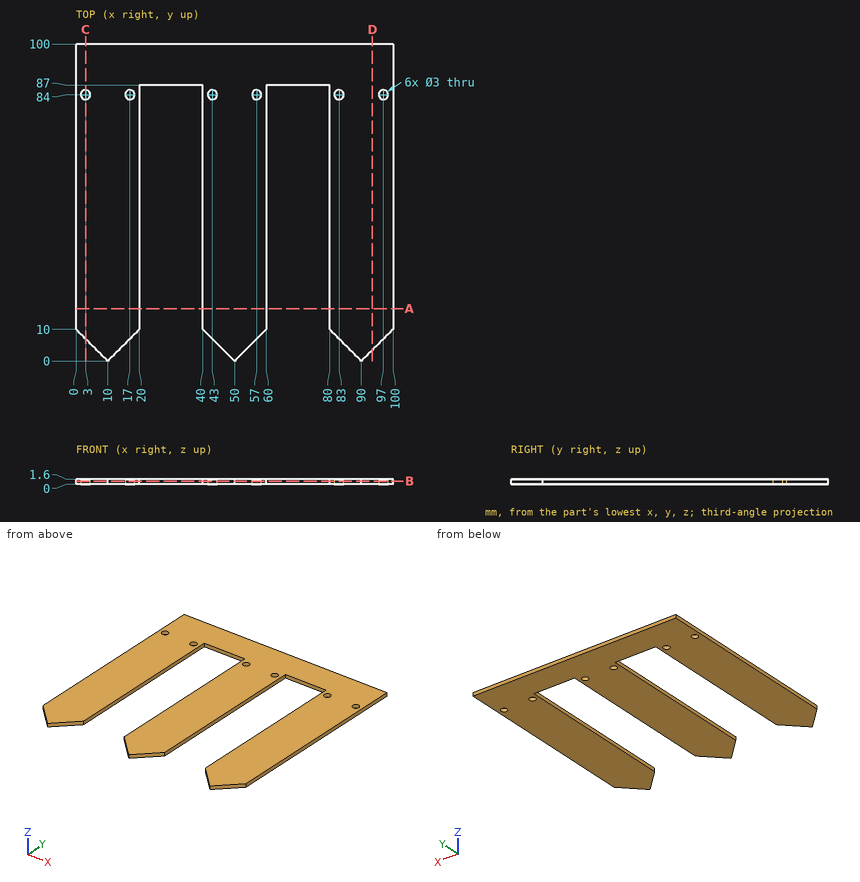
Geometry check sheet. Reference: drawing and pictorial views, mm from the part's lowest x, y, z. Round coordinates to 2 decimals unless told otherwise and drop trailing zeros. Order: outer loops, then holes, each group sorted by start corner. A loop starts at its lowest first (then second) coordinate and runs counter-clockwise, first axis right, second up. Notation, with made-up numbers: (25.25, -10) - (35.25, -10) arc R24 ccw to (35.25, 0) - close; hole circle Ø9 at (41.5, -29.75). An arc over 180 degrees is marked (long way). One line per question, with ' | ' between items. Start each with the question number.
(1) Sectioned sample at C-C on x = 3. Record the cut outline in (y, z), and give its area (3 significant figures).
(2) Sectioned sample at A-A on y = 16.5. Record the cut outline in (x, z).
(3) Depth check by flat-ended pin: pin 1 Ø0.5 at (x, z) = (32.5, 1) entering from -Y. Enter the tip coordinate at first touch or a pass-through.
(4) Sectioned sample at B-B on z = 0.9. Record the cut outline in (x, y).
(5) Thickness scan on L1, parallel to X at y = 37.5, z = 1; L2, parallel to X at y = 5, z = 0.6; L3, parallel to Y at x = 83, z = 1.2. Record the ranges inside material, lowest first. Write a range as [from, to].
(6) Sectioned sample at D-D on x = 93.5. Record the cut outline in (y, z), and give its area (3 significant figures).
Conclusion:
1) outline: (7, 0) - (82.5, 0) - (82.5, 1.6) - (7, 1.6) - close; (85.5, 0) - (100, 0) - (100, 1.6) - (85.5, 1.6) - close | area: 144 mm2
2) outline: (0, 0) - (20, 0) - (20, 1.6) - (0, 1.6) - close; (40, 0) - (60, 0) - (60, 1.6) - (40, 1.6) - close; (80, 0) - (100, 0) - (100, 1.6) - (80, 1.6) - close
3) pin 1: stops at y = 87
4) outline: (0, 10) - (10, 0) - (20, 10) - (20, 87) - (40, 87) - (40, 10) - (50, 0) - (60, 10) - (60, 87) - (80, 87) - (80, 10) - (90, 0) - (100, 10) - (100, 100) - (0, 100) - close; hole circle Ø3 at (3, 84); hole circle Ø3 at (17, 84); hole circle Ø3 at (43, 84); hole circle Ø3 at (57, 84); hole circle Ø3 at (83, 84); hole circle Ø3 at (97, 84)
5) L1: x = [0, 20], [40, 60], [80, 100] | L2: x = [5, 15], [45, 55], [85, 95] | L3: y = [7, 82.5], [85.5, 100]
6) outline: (3.5, 0) - (100, 0) - (100, 1.6) - (3.5, 1.6) - close | area: 154 mm2
